```python
from build123d import *

# Parameters (mm, degrees)
SKETCH2_R           = 32.9
SKETCH2_R_2         = 10.4
BOSS_EXTRUDE1_DEPTH = 25
SKETCH4_W           = 2.4
SKETCH4_H           = 20
CUT_EXTRUDE1_DEPTH  = 22
CUT_EXTRUDE2_DEPTH  = 1.5
SKETCH6_R           = 3.625
CUT_EXTRUDE3_DEPTH  = 3.25
FILLET1_R           = 0.75
CUT_EXTRUDE4_REACH  = 58.098
SKETCH7_R           = 2.625
CHAMFER1_SIZE       = 0.5
SKETCH8_R           = 1.5
CUT_EXTRUDE5_DEPTH  = 8.5
FILLET2_R           = 1.2


with BuildPart() as part:
    # Sketch2 → Boss-Extrude1 (new body)
    with BuildSketch(Plane.XY):
        with Locations((9.62, 10)):
            Circle(SKETCH2_R)
        with Locations((9.62, 10)):
            Circle(SKETCH2_R_2, mode=Mode.SUBTRACT)
    extrude(amount=BOSS_EXTRUDE1_DEPTH)

    # Sketch4 → Cut-Extrude1 (cut)
    with BuildSketch(Plane.XY.offset(25)):
        with BuildLine():
            Line((-11.82822809, -10.5), (17.12, -10.5))
            Line((17.12, -10.5), (17.12, -18.5))
            Line((17.12, -18.5), (26.056544649, -18.5))
            ThreePointArc((26.056544649, -18.5), (42.52, 10), (26.056544649, 38.5))
            Line((26.056544649, 38.5), (17.12, 38.5))
            Line((17.12, 38.5), (17.12, 30.5))
            Line((17.12, 30.5), (7.12, 30.5))
            Line((7.12, 30.5), (7.12, 34.339279361))
            ThreePointArc((7.12, 34.339279361), (5.349790899, 38.156143355), (1.292619701, 39.270348397))
            ThreePointArc((1.292619701, 39.270348397), (-4.45403874, 37.633425382), (-9.697773665, 34.768666365))
            ThreePointArc((-9.697773665, 34.768666365), (-11.263751051, 32.981913664), (-11.82822809, 30.674071368))
            Line((-11.82822809, 30.674071368), (-11.82822809, -10.5))
        make_face()
        with Locations((31.32, 0)):
            Rectangle(SKETCH4_W, SKETCH4_H, mode=Mode.SUBTRACT)
        with BuildLine():
            Line((-16.82822809, -9.567862195), (-16.82822809, 29.567862195))
            ThreePointArc((-16.82822809, 29.567862195), (-23.28, 10), (-16.82822809, -9.567862195))
        make_face()
    extrude(amount=-CUT_EXTRUDE1_DEPTH, mode=Mode.SUBTRACT)

    # Sketch5 → Cut-Extrude2 (cut)
    with BuildSketch(Plane.XY.offset(3)):
        with BuildLine():
            Line((17.12, 38.5), (26.056544649, 38.5))
            ThreePointArc((26.056544649, 38.5), (42.52, 10), (26.056544649, -18.5))
            Line((26.056544649, -18.5), (17.12, -18.5))
            Line((17.12, -18.5), (17.12, -10))
            Line((17.12, -10), (32.52, -10))
            Line((32.52, -10), (32.52, 10))
            Line((32.52, 10), (30.12, 10))
            Line((30.12, 10), (30.12, 30))
            Line((30.12, 30), (17.12, 30))
            Line((17.12, 30), (17.12, 38.5))
        make_face()
        with BuildLine():
            Line((-16.82822809, -9.567862195), (-16.82822809, 29.567862195))
            ThreePointArc((-16.82822809, 29.567862195), (-23.28, 10), (-16.82822809, -9.567862195))
        make_face()
    extrude(amount=-CUT_EXTRUDE2_DEPTH, mode=Mode.SUBTRACT)

    # Sketch6 → Cut-Extrude3 (cut)
    with BuildSketch(Plane.ZY.offset(16.82822809)):
        with Locations((13.1, 19.62)):
            Circle(SKETCH6_R)
    extrude(amount=-CUT_EXTRUDE3_DEPTH, mode=Mode.SUBTRACT)

    # Fillet1
    fillet1_edges = [part.edges().sort_by_distance(p)[0] for p in [
        (-16.82822809, 19.62, 9.475),
    ]]
    fillet(fillet1_edges, radius=FILLET1_R)

    # Sketch7 → Cut-Extrude4 (cut, up to next)
    with BuildSketch(Plane.ZY.offset(13.57822809), mode=Mode.PRIVATE) as cut_extrude4_sk1:
        with Locations((13.1, 19.62)):
            Circle(SKETCH7_R)
    cut_extrude4_tool1 = extrude(cut_extrude4_sk1.sketch, amount=-CUT_EXTRUDE4_REACH, mode=Mode.PRIVATE) & part.part
    add(cut_extrude4_tool1.solids().sort_by_distance((-13.578228, 19.62, 13.1))[0], mode=Mode.SUBTRACT)

    # Chamfer1
    chamfer1_edges = [part.edges().sort_by_distance(p)[0] for p in [
        (-13.57822809, 19.62, 10.475),
        (-11.82822809, 19.62, 10.475),
    ]]
    chamfer(chamfer1_edges, length=CHAMFER1_SIZE)

    # Sketch8 → Cut-Extrude5 (cut)
    with BuildSketch(Plane(origin=(17.12, 0, 0), x_dir=(0, 0, -1), z_dir=(1, 0, 0))):
        with Locations((-18.14, -15)):
            Circle(SKETCH8_R)
        with Locations((-8.06, -15)):
            Circle(SKETCH8_R)
        with Locations((-18.14, 35)):
            Circle(SKETCH8_R)
        with Locations((-8.06, 35)):
            Circle(SKETCH8_R)
    extrude(amount=-CUT_EXTRUDE5_DEPTH, mode=Mode.SUBTRACT)

    # Fillet2
    fillet2_edges = [part.edges().sort_by_distance(p)[0] for p in [
        (26.056544649, -18.5, 13.25),
        (26.056544649, 38.5, 13.25),
    ]]
    fillet(fillet2_edges, radius=FILLET2_R)


solid = part.part
```
Input: part model. Units: mm. Frame: model coordinates. A direction names the side the tool comes from. Give positions to 0.01 mm unless a question says otherwise; leave off trailing zeros. Order: outer loops, then holes, each group sorted by start corner. A loop starts at its lowest first (then second) coordinate and runs counter-clockwise, first axis right, second up.
1. Cut plane B-B (z = 13.1). State how many separate pieces and enclosed holes the cut face has, and give its area (3 significant figures).
Computed:
separate pieces: 3
enclosed holes: 0
area: 742 mm2
2. Cut plane C-C (y = 19.62). Return loops of the section in (x, z) (3 decimals).
Computed:
outline: (-21.842, 0) - (5.668, 0) - (5.668, 3) - (-11.828, 3) - (-11.828, 9.975) - (-12.328, 10.475) - (-13.078, 10.475) - (-13.578, 9.975) - (-13.578, 9.475) - (-16.078, 9.475) arc R0.75 ccw to (-16.828, 8.725) - (-16.828, 1.5) - (-21.842, 1.5) - close; (-16.828, 17.475) arc R0.75 ccw to (-16.078, 16.725) - (-13.578, 16.725) - (-13.578, 16.225) - (-13.078, 15.725) - (-12.328, 15.725) - (-11.828, 16.225) - (-11.828, 25) - (-16.828, 25) - close; (13.572, 0) - (41.082, 0) - (41.082, 1.5) - (30.12, 1.5) - (30.12, 3) - (13.572, 3) - close
3. Draft query along X for faces 4 (the face through (24, 30, 2)), 5 (the face through (8.62, -15, 18)), 6 (the face through (30.12, 0, 14)). Return one class per face: released by +X, released by -X, zero draft, split by the parting line, or undercut.
Computed:
face 4: zero draft
face 5: released by +X
face 6: undercut
4. Cut plane D-D (z = 23). Return loops of the section in (x, y).
Computed:
outline: (-16.83, -9.57) arc R32.9 ccw to (21.12, -20.82) arc R1.2 ccw to (20.7, -18.5) - (17.12, -18.5) - (17.12, -10.5) - (-11.83, -10.5) - (-11.83, 30.67) arc R5 cw to (-9.7, 34.77) arc R26.91 cw to (1.29, 39.27) arc R5 cw to (7.12, 34.34) - (7.12, 30.5) - (17.12, 30.5) - (17.12, 38.5) - (20.7, 38.5) arc R1.2 ccw to (21.12, 40.82) arc R32.9 ccw to (-16.83, 29.57) - close; (30.12, -10) - (32.52, -10) - (32.52, 10) - (30.12, 10) - close
5. Pin query (flat end, axial travel): pin 1 Ø10 at (x, y) = (7, 0) entering from -Z; pin 2 Ø2 at (y, z) = (18, 6) entering from +X; pin 3 Ø12 at (x, z) = (-4.5, 12.5) entering from +Y; pin 4 Ø12.5 at (x, z) = (27, 16.5) entering from -Y. Return the tip coordinate at first contact, or that it passes through.
Computed:
pin 1: stops at z = 0
pin 2: stops at x = -11.83
pin 3: stops at y = 41.88
pin 4: stops at y = -20.96
6. Cut plane A-A (x = 9.62). Return loops of the section in (y, z).
Computed:
outline: (-22.9, 0) - (-0.4, 0) - (-0.4, 3) - (-10.5, 3) - (-10.5, 25) - (-22.9, 25) - close; (20.4, 0) - (42.9, 0) - (42.9, 25) - (30.5, 25) - (30.5, 3) - (20.4, 3) - close; hole circle Ø3 at (-15, 8.06); hole circle Ø3 at (-15, 18.14); hole circle Ø3 at (35, 8.06); hole circle Ø3 at (35, 18.14)
7. Line query: probe 1 along X at (y, z) = (-1.5, 8.25); probe 2 along X at (y, z) = (10, 1.4); probe 3 along Y at (x, z) = (9.62, 2.4). Output: solid intervals per line, ascending.
Computed:
probe 1: x = -16.83 to -11.83, 30.12 to 32.52
probe 2: x = -23.28 to -0.78, 20.02 to 42.52
probe 3: y = -22.9 to -0.4, 20.4 to 42.9
8. Set-up query: faces 1 (the face through (21.878, -19.464, 13.414)), 2 (the face through (8.62, 35, 18)), 3 (the face through (32.52, 0, 13)). Return all of +Z, -Z, +X, -X, +Y, -Y with unobstructed straight access to the full face (end or side cutting, diameter ignored); none if empty.
Computed:
face 1: +Z, +X
face 2: +X
face 3: +Z, +X, +Y, -Y
